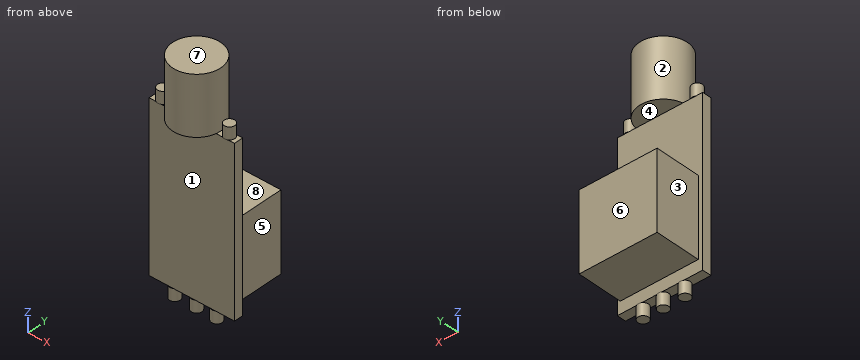
Autodesk Inventor part; units mm, degrees
ref_plane "YZ Plane" through (0, 0, 0) normal (1, 0, 0) x (0, 1, 0)
ref_plane "XZ Plane" through (0, 0, 0) normal (0, 1, 0) x (-1, 0, 0)
ref_plane "XY Plane" through (0, 0, 0) normal (0, 0, 1) x (1, 0, 0)
sketch "Sketch1" plane through (0, 0, 0) normal (0, 1, 0) x (-1, 0, 0)
  line L0 (16.1537, 17.2566) -> (-1.9057, 17.2566)
  line L1 (-1.9057, 17.2566) -> (-1.9057, -17.516)
  line L2 (-1.9057, -17.516) -> (16.1537, -17.516)
  line L3 (16.1537, -17.516) -> (16.1537, 17.2566)
  point P0 (0, 0)
  dimension "d0" = 34.7726
  dimension "d1" = 18.0594
extrude "Extrusion1" add sketch "Sketch1" along normal blind 1.9304
sketch "Sketch2" plane through (0, 1.9304, 0) normal (0, 1, 0) x (1, 0, 0)
  line L0 (-15.2139, -1.4832) -> (1.2961, -1.4832)
  line L1 (1.2961, -1.4832) -> (1.2961, 14.976)
  line L2 (1.2961, 14.976) -> (-15.2139, 14.976)
  line L3 (-15.2139, 14.976) -> (-15.2139, -1.4832)
  line L4 (1.9057, -17.2566) -> (1.9057, 17.516)
  line L5 (1.9057, 17.516) -> (-16.1537, 17.516)
  line L6 (-16.1537, -17.2566) -> (1.9057, -17.2566)
  point P0 (0, 0)
  dimension "d4" = 16.4592
  dimension "d5" = 16.51
  dimension "d6" = 0.6096
  dimension "d9" = 15.7734
extrude "Extrusion2" add sketch "Sketch2" along normal blind 9.6774
sketch "Sketch3" plane through (-16.1537, 0, 17.2566) normal (0, 0, 1) x (1, 0, 0)
  line L0 (17.4498, 1.9304) -> (0.9398, 1.9304)
  line L1 (9.1948, 1.9304) -> (9.1948, -4.4517)
  line L2 (18.0594, 0) -> (18.0594, 1.9304)
  line L3 (18.0594, 0.9652) -> (-4.716, 0.9652)
  circle A0 centre (9.1948, 0.9652) radius 5.08
  point P0 (16.1537, 0)
  dimension "d12" = 10.16
extrude "Extrusion3" add sketch "Sketch3" along normal blind 12.3444
sketch "Sketch4" plane through (1.9057, 0, -17.516) normal (0, 0, -1) x (-1, 0, 0)
  line L0 (0, 0) -> (0, 1.9304)
  line L1 (0, 0.9652) -> (18.0594, 0.9652)
  line L2 (18.0594, 0) -> (18.0594, 1.9304)
  line L3 (13.8521, 1.9304) -> (3.8771, 1.9304)
  line L4 (8.8646, 1.9304) -> (8.8646, -5.2451)
  line L5 (18.0594, 1.3992) -> (13.462, 1.3992)
  line L6 (13.462, 1.9304) -> (13.462, -4.7459)
  line L7 (0, 1.6034) -> (4.5974, 1.6034)
  line L8 (4.5974, 1.9304) -> (4.5974, -5.3585)
  circle A0 centre (4.5974, 0.9652) radius 1.1176
  circle A1 centre (8.8646, 0.9652) radius 1.1176
  circle A2 centre (13.462, 0.9652) radius 1.1176
  point P0 (1.9057, 0)
  dimension "d15" = 9.1948
  dimension "d16" = 4.5974
  dimension "d17" = 4.5974
  dimension "d18" = 2.2352
  dimension "d19" = 2.2352
  dimension "d20" = 2.2352
extrude "Extrusion4" add sketch "Sketch4" along normal blind 2.54 contours A0 L7 L8 L1 | L1 L8 A0 | A0 L3 L8 L7 | L8 L3 A0 L1 | L1 A0 L8 | A0 L3 | A1 L3 L4 L1 | L1 L4 A1 | A1 L3 | L4 L3 A1 L1 | L1 A1 L4 | A2 L5 L6 L3 | L3 L6 L1 A2 | L1 L6 A2 | A2 L1 L6 L5 | L1 A2 L6
sketch "Sketch5" plane through (1.9057, 0, 17.2566) normal (0, 0, 1) x (1, 0, 0)
  circle A0 centre (-1.9057, 0.9652) radius 1.1147
  circle A1 centre (-16.0424, 0.9652) radius 1.1215
  point P0 (-1.9057, 0)
extrude "Extrusion5" add sketch "Sketch5" along normal blind 2.54
equation "\"d19\" = d18"
equation "\"d20\" = d18"
properties part number "Motor Driver"
Work out the finished part from the listing and answer in its coordinate system (mm). Face numbers are marked on the shaded views. A direction names the side the tool comes from. Round coordinates to 2 decimals unless told otherwise and drop trailing zeros. Loops run counter-clockwise (first coordinate to the right, second up) from the corner with the lowest first, then second, coordinate; pieces in that order, holes last. Notation, with made-up numbers: M 17,42.25 L 68,42.25 A14 ccw 68,49.25 Z; hole C 26,4.25 d6. An arc over 180 degrees is marked long. Use CSV: the item, a comma, the result in double quotes.
Q1. Section C-C, the plane y = 8 is taken. Determine the outline of the cut face in (x, z).
Determined:
outline,"M -15.21,-14.98 L 1.3,-14.98 L 1.3,1.48 L -15.21,1.48 Z"
Q2. Each of these flat-tipped pins is pushed along its axis until it touches: pin 1 (0.6 mm diameter, centred on x = -13.5, y = 0.5, fed in from -Z); pin 2 (8 mm diameter, centred on x = -8.5, y = 9.5, fed in from +Z); pin 3 (6 mm diameter, centred on y = 9, z = 0, fed in from +X); pin 4 (6 mm diameter, centred on y = 8.5, z = 24, fed in from -X). Where does it stop, or does it pass through?
Determined:
pin 1,"z = -17.52"
pin 2,"z = 29.6"
pin 3,"x = 1.3"
pin 4,"x = -9.25"
Q3. Section A-A, the plane x = 0 is taken. Determine the outline of the cut face in (y, z).
Determined:
outline,"M -0.15,17.26 L 0,17.26 L 0,-17.52 L 1.93,-17.52 L 1.93,-14.98 L 11.61,-14.98 L 11.61,1.48 L 1.93,1.48 L 1.93,17.26 L 2.08,17.26 L 2.08,19.8 L -0.15,19.8 Z"
Q4. Section D-D, the plane z = 21 is taken. Determine the outline of the cut face in (x, y), then the cut area to 3 significant figures.
Determined:
outline,"C -6.96,0.97 d10.16"
area,"81.1 mm2"
Q5. The mould has two halves that part along Z. Classify the marked faces 6, 7 and 8: pulls with the +Z half, pulls with the -Z half, needs draft (parallel to the pull), parting line crosses it, or undercut.
Determined:
face 6,"needs draft"
face 7,"pulls with the +Z half"
face 8,"undercut"
Q6. A tool of negligible diameter and unlimited length cuts with its end or side. For the marked faces 1, 2, 3, 4 and 5, from which of +Z, -Z, +X, -X, +Y, -Y can it reach the whole face along a straight path? Write none if from no direction.
Determined:
face 1,"+X, -X, -Y"
face 2,"+Z"
face 3,"+Z, -Z, -X, +Y"
face 4,"+X, -X, +Y"
face 5,"+Z, -Z, +X, +Y"
Q7. Consider L1, parallel to Z at x = -12.25, y = 2; L2, parallel to Z at x = -11.25, y = -1; L3, parallel to Y at x = -15, z = 10. Determine where each line is inside the solid, lowest interval first.
Determined:
L1,"-14.98 to 1.48"
L2,"17.26 to 29.6"
L3,"0 to 1.93"
Q8. Section B-B, the plane z = -8 is taken. Determine the outline of the cut face in (x, y), then the cut area to 3 significant figures.
Determined:
outline,"M -16.15,0 L 1.91,0 L 1.91,1.93 L 1.3,1.93 L 1.3,11.61 L -15.21,11.61 L -15.21,1.93 L -16.15,1.93 Z"
area,"195 mm2"
